Here's how the part is built. I have some questions about the finished solid (model axes, mm). A direction names the side the tool comes from. Round coordinates to 2 decimals unless told otherwise and drop trailing zeros. Order: outer loops, then holes, each group sorted by start corner. A loop starts at its lowest first (then second) coordinate and runs counter-clockwise, first axis right, second up. Notation, with made-up numbers: M -34,69 L 13,69 A17 cw 13,75 Z; hole C 35.25,21.25 d7. An arc over 180 degrees is marked long. Write each question's results on one line, items separated by ' | '. Start each with the question number.
```python
from build123d import *

# Parameters (mm, degrees)
F0_R     = 2.5
F1_DEPTH = 12
F3_R     = 1.25


with BuildPart() as f1:
    # F0 (on Front) → F1 (new body)
    with BuildSketch(Plane.XZ):
        Circle(F0_R)
    extrude(amount=-F1_DEPTH)

    # F4: sweep along a path in F2
    with BuildLine(Plane.YZ) as f4_path:
        Line((12, 0), (22, 0))
        ThreePointArc((22, 0), (24.1213203436, -0.8786796564), (25, -3))
        Line((25, -3), (25, -13))
    # F3 (on face) → F4 (sweep)
    with BuildSketch(Plane(origin=(0, 12, 0), x_dir=(-1, 0, 0), z_dir=(0, 1, 0))):
        Circle(F3_R)
    sweep(path=f4_path.line)


solid = f1.part
```
(1) On a 3-axis mill with a long thin cutter (end or side, diameter ignored), from which of +Z, -Z, +X, -X, +Y, -Y can I reach the whole of each face in a straight line? I mean faces 1 (the cylindrical face through (0.27, 23.78, -8.07)), 2 (the flat face through (0, 25, -13)). Say none if no direction works.
(2) I want a section at A-A on x = 0. Write out the boundary of the cut face in (y, z).
(3) I want a section at B-B on y = 14.25. Write out the boundary of the cut face in (x, z).
(4) I want a section at C-C on z = -10.5. Write out the boundary of the cut face in (x, y).
(5) I want a section at D-D on x = 1.5. Write out the boundary of the cut face in (y, z).
(6) I'm going to push flat-ended pins straight in: pin 1 Ø4 at (y, z) = (9.5, -3.5) entering from -X; pin 2 Ø1.5 at (x, z) = (-0.5, 0.5) entering from +Y; pin 3 Ø5 at (y, z) = (10.5, -3.5) entering from +X. Where does each tip first touch, or does it pass through?
(7) If we mould it in two halves opening along Y, with no side actions, what happens to faces 3 (the cylindrical face through (-0.54, 5.92, -2.44)), 4 (the cylindrical face through (0.27, 17.07, -1.22)), 5 (the flat face through (0, 0, 0)), 6 (the flat face through (-1, 12, -1))? For each: pulls with the +Y half, pulls with the -Y half, needs draft (parallel to the pull), parting line crosses it, or undercut.
(8) Please list where these lines run through material, in increasing order: line 1 (Y direction, x = -0.8, z = 2); line 2 (Z direction, x = 0.65, y = 5); line 3 (Z direction, x = 0.8, y = 22.5).
Solutions:
1) face 1: -Z | face 2: -Z, +X, -X, +Y, -Y
2) outline: M 0,-2.5 L 12,-2.5 L 12,-1.25 L 22,-1.25 A1.75 cw 23.75,-3 L 23.75,-13 L 26.25,-13 L 26.25,-3 A4.25 ccw 22,1.25 L 12,1.25 L 12,2.5 L 0,2.5 Z
3) outline: C 0,0 d2.5
4) outline: C 0,25 d2.5
5) outline: M 0,-2 L 12,-2 L 12,2 L 0,2 Z
6) pin 1: x = -2 | pin 2: y = 25.17 | pin 3: x = 2.29
7) face 3: needs draft | face 4: undercut | face 5: pulls with the -Y half | face 6: undercut
8) line 1: 0 to 12 | line 2: -2.41 to 2.41 | line 3: -1.02 to 0.93
